The model under review builds one solid part; all positions refer to its coordinate system, in mm. Face numbers are marked on the shaded views. Give positions to 0.01 mm unless a question says otherwise; leave off trailing zeros. Loops run counter-clockwise (first coordinate to the right, second up) from the corner with the lowest first, then second, coordinate; pieces in that order, holes last. Notation, with made-up numbers: M 76.25,10.5 L 132.25,10.5 A22 ccw 132.25,37.5 Z; hole C -6,46 d7. An arc over 180 degrees is marked long. One line per item, written item: value. Start each with the question number.
Q1. Mouldability with a two-part tool opening along X and no side actions: class the marked faces 1, 2 and 3 as released by +X, released by -X, zero draft, split by the parting line, or undercut.
Q2. We need section A-A on x = 0. Write out the cut boundary in (y, z), plus the area to 3 significant figures.
Q3. We need section B-B on y = 14. Write out the cut boundary in (x, z).
Q4. We need section D-D on x = -9. Write out the cut boundary in (y, z).
Q5. We need section C-C on z = -3.75. Write out the cut boundary in (x, y), plus the area to 3 significant figures.
Q6. To check wall thickness, follow line 1 along X through (y, z) = (11, -10.25); line 2 along X through (y, z) = (46, -7); line 3 along Y through (x, z) = (8, -7.5). State the ranges of each line that lie inside material, in increasing order. Write a range as from..to.
Q7. For pin 1 (6 mm diameter, centred on x = 12, z = -3.5, fed in from +Y); pin 2 (6 mm diameter, centred on x = -11, y = 11, fed in from -Z), all flat-tipped, find the tip position at first contact; note any pin that passes through.
Autodesk Inventor part; units mm, degrees
ref_plane "to_bearing_XY" through (0, 46, -6.5) normal (0, 0, 1) x (1, 0, 0)
ref_plane "to_bearing_YZ" through (0, 46, -6.5) normal (1, 0, 0) x (0, 1, 0)
ref_plane "to_bearing_ZX" through (0, 46, -6.5) normal (0, 1, 0) x (0, 0, 1)
sketch "Sketch_7" plane through (0, 0, 0) normal (0, 0, 1) x (1, 0, 0)
  line L0 (-25, 46) -> (-25, 0)
  line L1 (-25, 0) -> (25, 0)
  line L2 (25, 0) -> (25, 46)
  arc A0 (25, 46) -> (-25, 46) centre (0, 46) ccw
extrude "Extrusion1" add sketch "Sketch_7" against normal blind 15
sketch "Sketch_8" plane through (0, 0, 0) normal (1, 0, 0) x (0, 0, -1)
  line L0 (15, 46) -> (2, 46)
  line L1 (2, 46) -> (2, 64.5)
  line L2 (2, 64.5) -> (11, 64.5)
  line L3 (11, 64.5) -> (11, 65.5)
  line L4 (11, 65.5) -> (12.5, 65.5)
  line L5 (12.5, 65.5) -> (12.5, 64.5)
  line L6 (12.5, 64.5) -> (15, 64.5)
  line L7 (15, 64.5) -> (15, 46)
  line L8 (15, 46) -> (2, 46)
revolve "Revolution1" cut sketch "Sketch_8" angle 360 about axis through (0, 46, -15) along (0, 0, -1)
sketch "Sketch_1" plane through (0, 0, 0) normal (1, 0, 0) x (0, 0, -1)
  line L0 (15, 46) -> (0, 46)
  line L1 (0, 46) -> (0, 63)
  line L2 (0, 63) -> (15, 63)
  line L3 (15, 63) -> (15, 46)
  line L4 (15, 46) -> (0, 46)
revolve "Revolution2" cut sketch "Sketch_1" angle 360 about axis through (0, 46, -15) along (0, 0, -1)
sketch "Sketch4" plane through (0, 0, -15) normal (0, 0, -1) x (-1, 0, 0)
  point P0 (11, 11)
hole "Hole1" at (-11, 11, -15) direction (0, 0, 1) diameter 10 depth 15
pattern_linear "Rectangular Pattern1" count 2 spacing 22 along (1, 0, 0) of "Hole1"
ref_plane "to_bearing_XY" through (0, 46, -6.5) normal (0, 0, 1) x (1, 0, 0)
ref_plane "to_bearing_YZ" through (0, 46, -6.5) normal (1, 0, 0) x (0, 1, 0)
ref_plane "to_bearing_ZX" through (0, 46, -6.5) normal (0, 1, 0) x (0, 0, 1)
ref_plane "to_retaining_ring_XY" through (0, 46, -12.5) normal (0, 0, -1) x (1, 0, 0)
ref_plane "to_retaining_ring_YZ" through (0, 46, -12.5) normal (1, 0, 0) x (0, -1, 0)
ref_plane "to_retaining_ring_ZX" through (0, 46, -12.5) normal (0, -1, 0) x (0, 0, -1)
properties part number "SBGSMA6904ZZ-35_h"
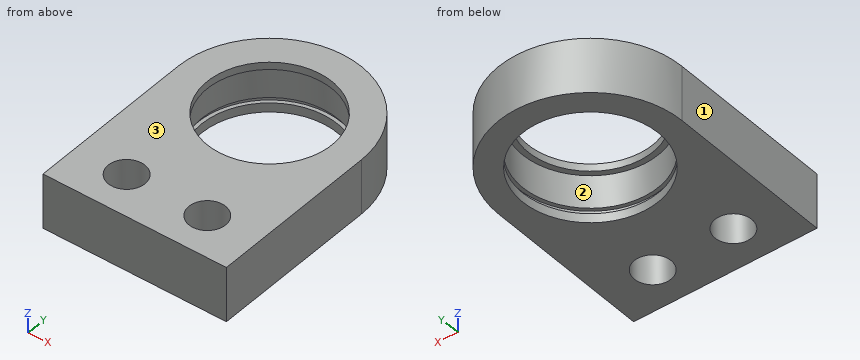
Solved:
1. face 1: released by -X
1. face 2: undercut
1. face 3: zero draft
2. outline: M 0,-15 L 27.5,-15 L 27.5,-12.5 L 26.5,-12.5 L 26.5,-11 L 27.5,-11 L 27.5,-2 L 29,-2 L 29,0 L 0,0 Z; M 63,-2 L 64.5,-2 L 64.5,-11 L 65.5,-11 L 65.5,-12.5 L 64.5,-12.5 L 64.5,-15 L 71,-15 L 71,0 L 63,0 Z
2. area: 513 mm2
3. outline: M -25,-15 L -15,-15 L -15,0 L -25,0 Z; M -7,-15 L 7,-15 L 7,0 L -7,0 Z; M 15,-15 L 25,-15 L 25,0 L 15,0 Z
4. outline: M 0,-15 L 6.42,-15 L 6.42,0 L 0,0 Z; M 15.58,-15 L 29.84,-15 L 29.84,-12.5 L 28.7,-12.5 L 28.7,-11 L 29.84,-11 L 29.84,-2 L 31.58,-2 L 31.58,0 L 15.58,0 Z; M 60.42,-2 L 62.16,-2 L 62.16,-11 L 63.3,-11 L 63.3,-12.5 L 62.16,-12.5 L 62.16,-15 L 69.32,-15 L 69.32,0 L 60.42,0 Z
5. outline: M -25,0 L 25,0 L 25,46 A25 ccw -25,46 Z; hole C 0,46 d37; hole C -11,11 d10; hole C 11,11 d10
5. area: 2,050 mm2
6. line 1: -25..-16, -6..6, 16..25
6. line 2: -25..-18.5, 18.5..25
6. line 3: 0..7, 15..29.32, 62.68..69.69
7. pin 1: y = 69.32
7. pin 2: through
